CAD build for the part. Positions are in the model's coordinates, mm. Face numbers are marked on the shaded views. A direction names the side the tool comes from. Round coordinates to 2 decimals unless told otherwise and drop trailing zeros. Loops run counter-clockwise (first coordinate to the right, second up) from the corner with the lowest first, then second, coordinate; pieces in that order, holes last.
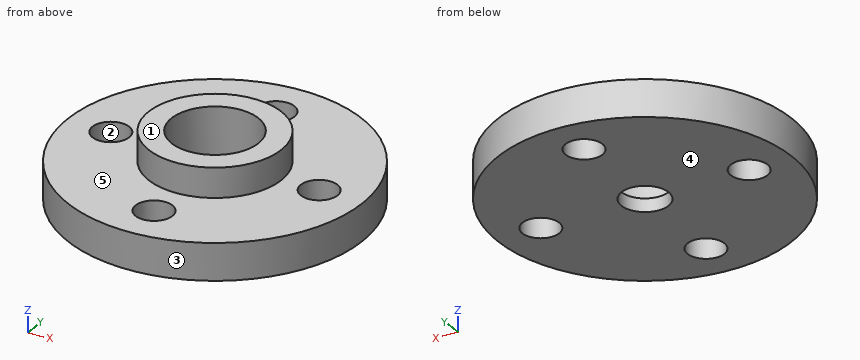
Autodesk Inventor part; units mm, degrees
ref_plane "YZ Plane" through (0, 0, 0) normal (1, 0, 0) x (0, 1, 0)
ref_plane "XZ Plane" through (0, 0, 0) normal (0, 1, 0) x (-1, 0, 0)
ref_plane "XY Plane" through (0, 0, 0) normal (0, 0, 1) x (1, 0, 0)
sketch "スケッチ1" plane through (0, 0, 0) normal (0, 0, 1) x (1, 0, 0)
  circle A0 centre (0, 0) radius 9.975
  dimension "d0" = 19.95
extrude "押し出し1" add sketch "スケッチ1" along normal blind 2.5
sketch "スケッチ2" plane through (0, 0, 2.5) normal (0, 0, 1) x (1, 0, 0)
  circle A0 centre (0, 0) radius 4.5
  dimension "d3" = 9
extrude "押し出し2" add sketch "スケッチ2" along normal blind 2
sketch "スケッチ3" plane through (0, 0, 4.5) normal (0, 0, 1) x (1, 0, 0)
  point P0 (0, 0)
  point P1 (0, 0)
hole "穴1" at (0, 0, 4.5) direction (0, 0, -1) diameter 3.2 end through all
sketch "スケッチ4" plane through (0, 0, 0) normal (0, 0, -1) x (-1, 0, 0)
  circle A0 centre (0, 0) radius 1.6 construction
  circle A1 centre (0, 0) radius 7 construction
  point P0 (7, 0)
  dimension "d13" = 14
hole "穴2" at (-7, 0, 0) direction (0, 0, 1) diameter 2.5 end through all
thread "ねじ1"
pattern_circular "円形状パターン1" count 4 over 360 about axis through (0, 0, -10) along (0, 0, 1) of "穴2"
sketch "スケッチ5" plane through (0, 0, 4.5) normal (0, 0, 1) x (1, 0, 0)
  circle A0 centre (0, 0) radius 2.95
  dimension "d26" = 5.9
extrude "押し出し3" cut sketch "スケッチ5" against normal blind 3.6
properties part number "feetech_servo-hone"
Item 1: Flat gauge pins, fed straight in: P1, Ø1.5, axis at x = 1, y = -4.5, coming from the -Z side; P2, Ø4, axis at x = 0, y = 0, coming from the +Z side; P3, Ø1, axis at x = 6.5, z = 2.5, coming from the -Y side; P4, Ø2, axis at y = -2.5, z = 3, coming from the +X side. Where does each tip first touch, or does it go through?
Answers follow:
P1: stops at z = 0
P2: stops at z = 0.9
P3: stops at y = -7.97
P4: stops at x = 9.84
Item 2: Cut at B-B, the plane x = -7. Give the cut face in (y, z), plus the area to 3 significant figures.
Answers follow:
outline: (-7.11, 0) - (-1.25, 0) - (-1.25, 2.5) - (-7.11, 2.5) - close; (1.25, 0) - (7.11, 0) - (7.11, 2.5) - (1.25, 2.5) - close
area: 29.3 mm2
Item 3: Cut at D-D, the plane y = -7.25. Give the cut face in (x, z), plus the area to 3 significant figures.
Answers follow:
outline: (-6.85, 0) - (-1.22, 0) - (-1.22, 2.5) - (-6.85, 2.5) - close; (1.22, 0) - (6.85, 0) - (6.85, 2.5) - (1.22, 2.5) - close
area: 28.1 mm2
Item 4: Cut at C-C, the plane x = 1. Give the cut face in (y, z).
Answers follow:
outline: (-9.92, 0) - (-7.75, 0) - (-7.75, 2.5) - (-9.92, 2.5) - close; (-6.25, 0) - (-1.25, 0) - (-1.25, 0.9) - (-2.78, 0.9) - (-2.78, 4.5) - (-4.39, 4.5) - (-4.39, 2.5) - (-6.25, 2.5) - close; (1.25, 0) - (6.25, 0) - (6.25, 2.5) - (4.39, 2.5) - (4.39, 4.5) - (2.78, 4.5) - (2.78, 0.9) - (1.25, 0.9) - close; (7.75, 0) - (9.92, 0) - (9.92, 2.5) - (7.75, 2.5) - close
Item 5: Cut at A-A, the plane y = 0. Give the cut face in (x, z) (3 decimals).
Answers follow:
outline: (-9.975, 0) - (-8.25, 0) - (-8.25, 2.5) - (-9.975, 2.5) - close; (-5.75, 0) - (-1.6, 0) - (-1.6, 0.9) - (-2.95, 0.9) - (-2.95, 4.5) - (-4.5, 4.5) - (-4.5, 2.5) - (-5.75, 2.5) - close; (1.6, 0) - (5.75, 0) - (5.75, 2.5) - (4.5, 2.5) - (4.5, 4.5) - (2.95, 4.5) - (2.95, 0.9) - (1.6, 0.9) - close; (8.25, 0) - (9.975, 0) - (9.975, 2.5) - (8.25, 2.5) - close
Item 6: Probe line 1 (Y direction, x = 0, z = 0.6) (3 decimals); line 2 (Y direction, x = 0, z = 1.3) (3 decimals); line 3 (Z direction, x = -5, y = -4.5). List the from-to ranges inside material, lowest first.
Answers follow:
line 1: y = -9.975 to -8.25, -5.75 to -1.6, 1.6 to 5.75, 8.25 to 9.975
line 2: y = -9.975 to -8.25, -5.75 to -2.95, 2.95 to 5.75, 8.25 to 9.975
line 3: z = 0 to 2.5
Item 7: Two-plate mould, pull along Y, no slides. Class the marked faces 1, 2 and 3: released by +Y, released by -Y, zero draft, split by the parting line, or undercut.
Answers follow:
face 1: zero draft
face 2: undercut
face 3: split by the parting line
Item 8: 3-axis set-ups, long thin cutter, end or side, ignore diameter. For the marked faces 4 and 5: which of +Z, -Z, +X, -X, +Y, -Y reach the whole face in a straight line?
Answers follow:
face 4: -Z, +X, -X, +Y, -Y
face 5: +Z
